Here's how the part is built. I have some questions about the finished solid (model axes, mm). A direction names the side the tool comes from. Round coordinates to 2 decimals unless told otherwise and drop trailing zeros. Loops run counter-clockwise (first coordinate to the right, second up) from the corner with the lowest first, then second, coordinate; pieces in that order, holes last. Notation, with made-up numbers: (-20, 14) -> (29, 14) arc R17 ccw to (29, 32) -> close; hole circle Ø1 at (-4, -24.75). An arc over 180 degrees is marked (long way). One line per item, written item: value. Start each with the question number.
```python
from build123d import *

# Parameters (mm, degrees)
EXTRUDE053_DEPTH               = 6
EXTRUDE053_PLACEMENT_ANGLE     = 180
CYLINDER127_R                  = 1.6
CYLINDER127_DEPTH              = 40
CYLINDER124_R                  = 1.6
CYLINDER124_DEPTH              = 40
EXTRUDE050_DEPTH               = 10
EXTRUDE049_DEPTH               = 21
PART_MIRRORING_PLACEMENT_ANGLE = 180


with BuildPart() as extrude053:
    # Sketch043 → Extrude053 (new body)
    with BuildSketch(Plane.XY):
        Polygon((-6.704267, 10), (14.295733, 10), (14.295733, 8.4), (13.295733, 8.4), (13.295733, 9.4), (12.295733, 9.4), (12.295733, 8.4), (11.295733, 8.4), (11.295733, 9.4), (10.295733, 9.4), (10.295733, 8.4), (9.295733, 8.4), (9.295733, 9.4), (8.295733, 9.4), (8.295733, 8.4), (7.295733, 8.4), (7.295733, 9.4), (6.295733, 9.4), (6.295733, 8.4), (5.295733, 8.4), (5.295733, 9.4), (4.295733, 9.4), (4.295733, 8.4), (3.295733, 8.4), (3.295733, 9.4), (2.295733, 9.4), (2.295733, 8.4), (1.295733, 8.4), (1.295733, 9.4), (0.295733, 9.4), (0.295733, 8.4), (-0.704267, 8.4), (-0.704267, 9.4), (-1.704267, 9.4), (-1.704267, 8.4), (-2.704267, 8.4), (-2.704267, 9.4), (-3.704267, 9.4), (-3.704267, 8.4), (-4.704267, 8.4), (-4.704267, 9.4), (-5.704267, 9.4), (-5.704267, 8.4), (-6.704267, 8.4), align=None)
    extrude(amount=EXTRUDE053_DEPTH)


with BuildPart() as extrude053_1:
    # Extrude053 placement: moved
    add(extrude053.part.moved(Location((9, 18.5, 43.9))).rotate(Axis((9, 18.5, 43.9), (0, 0, 1)), EXTRUDE053_PLACEMENT_ANGLE))


with BuildPart() as cylinder127:
    # Cylinder127 → Cylinder127 (new body)
    with BuildSketch(Plane(origin=(5.3, 42, 40.5), x_dir=(0, 0, -1), z_dir=(0, -1, 0))):
        Circle(CYLINDER127_R)
    extrude(amount=CYLINDER127_DEPTH)


with BuildPart() as cylinder124:
    # Cylinder124 → Cylinder124 (new body)
    with BuildSketch(Plane(origin=(8.3, 42, 54.5), x_dir=(0, 0, -1), z_dir=(0, -1, 0))):
        Circle(CYLINDER124_R)
    extrude(amount=CYLINDER124_DEPTH)


with BuildPart() as extrude050:
    # Sketch040 → Extrude050 (new body)
    with BuildSketch(Plane.XZ):
        Polygon((-8.16038, 62.64716), (-8.16038, 30.419451), (4.410427, 62.64716), align=None)
    extrude(amount=-EXTRUDE050_DEPTH)


with BuildPart() as extrude050_1:
    # Extrude050 placement: moved
    add(extrude050.part.moved(Location((0, 8, 0))))


with BuildPart() as cut132:
    # Sketch039 → Extrude049 (new body)
    with BuildSketch(Plane.YZ):
        Polygon((8.5, 62), (8.5, 35), (12.616711, 35), (14.5, 62), align=None)
    extrude(amount=EXTRUDE049_DEPTH)


with BuildPart() as cut132_1:
    # Extrude049 placement: moved
    add(cut132.part.moved(Location((-7, 0, 0))))

    # Cut127: cut Extrude050
    add(extrude050_1.part, mode=Mode.SUBTRACT)

    # Cut130: cut Cylinder124
    add(cylinder124.part, mode=Mode.SUBTRACT)

    # Cut131: cut Cylinder127
    add(cylinder127.part, mode=Mode.SUBTRACT)

    # Cut132: cut Extrude053
    add(extrude053_1.part, mode=Mode.SUBTRACT)


with BuildPart() as part_mirroring:
    # Part__Mirroring: instance of Cut132
    add(cut132_1.part.mirror(Plane(origin=(3.813159, 4e-06, 48.5), x_dir=(1, 0, 0), z_dir=(0, 1, 0))))


with BuildPart() as part_mirroring_1:
    # Part__Mirroring placement: moved
    add(part_mirroring.part.moved(Location((237.8, 0, 0))).rotate(Axis((237.8, 0, 0), (0, 0, 1)), PART_MIRRORING_PLACEMENT_ANGLE))


solid = part_mirroring_1.part
```
Q1. If we mould it in two halves opening along X, with no side actions, what happens to faces 1 (the flat face through (230.096, 9.6, 46.9)), 2 (the flat face through (234, 11, 35)), 3 (the flat face through (240.096, 9.6, 44.7)), 4 (the flat face through (223.8, 11, 49))? For each: released by +X, released by -X, zero draft, split by the parting line, or undercut.
Q2. Which directions (+Z, -Z, +X, -X, +Y, -Y) give clear straight access to the entire face, cutting with the end or side of a thin tool? Please do faces 5 (the flat face through (239.096, 9.6, 45.9)), 6 (the cylindrical face through (228.15, 11.34, 53.64)), 7 (the flat face through (225.6, 9.1, 46.9)), 8 (the flat face through (226.6, 10.1, 46.9)).
Q3. I want a section at A-A on x = 228.5. Please give me the cut outline in (y, z).
Q4. I want a section at B-B on z = 54.5. Please give me the cut outline in (x, y).
Q5. I want a section at D-D on y = 13.5. Please give me the cut outline in (x, z).
Q6. I want a section at C-C on y = 12. Please give me the cut outline in (x, z).
Q7. Will these pins go through, and if not, where does the flat tip stop? P1, Ø0.8, axis at y = 9.5, z = 47.5, coming from the +X side; P2, Ø0.5, axis at y = 9.5, z = 48.5, coming from the +X side; P3, Ø5, axis at x = 229.5, z = 54.5, coming from the +Y side.
Q8. If I drill on line 1 along Z through (x, y) = (232.5, 10.55); line 2 along Y through (x, z) = (234.5, 56); line 3 along X through (y, z) = (10.5, 54.5), over which ranges is the centre line in solid material (lowest first)?
Answers below:
1. face 1: undercut
1. face 2: zero draft
1. face 3: released by +X
1. face 4: released by -X
2. face 5: +Z, -Y
2. face 6: +Y, -Y
2. face 7: +X, -X, -Y
2. face 8: -Y
3. outline: (8.5, 35) -> (12.62, 35) -> (13.89, 53.25) -> (8.5, 53.25) -> (8.5, 49.9) -> (10.1, 49.9) -> (10.1, 43.9) -> (8.5, 43.9) -> close; (8.5, 55.75) -> (14.06, 55.75) -> (14.5, 62) -> (8.5, 62) -> close
4. outline: (223.8, 8.5) -> (227.9, 8.5) -> (227.9, 13.98) -> (223.8, 13.98) -> close; (231.1, 8.5) -> (236.57, 8.5) -> (236.57, 13.98) -> (231.1, 13.98) -> close
5. outline: (223.8, 47.66) -> (239.23, 47.66) -> (233.64, 62) -> (223.8, 62) -> close; hole circle Ø3.2 at (229.5, 54.5)
6. outline: (223.8, 35) -> (244.17, 35) -> (233.64, 62) -> (223.8, 62) -> close; hole circle Ø3.2 at (229.5, 54.5); hole circle Ø3.2 at (232.5, 40.5)
7. P1: stops at x = 239.45
7. P2: stops at x = 238.1
7. P3: stops at y = 14.15
8. line 1: z = 35 to 38.9, 42.1 to 62
8. line 2: y = 8.5 to 14.08
8. line 3: x = 223.8 to 227.9, 231.1 to 236.57
